Read the model definition and answer for the solid it produces. Units are mm, in the model's axes. A direction names the side the tool comes from. Give positions to 0.01 mm unless a question says otherwise; leave off trailing zeros. Write each loop counter-clockwise with the first axis right and the second up, starting at its lowest first coordinate (ties: lowest second). Pieces come first, ordered by that corner, then holes. Notation, with made-up numbers: (4.25, -38.5) -> (45.25, -38.5) arc R19 ccw to (45.25, -6.5) -> close; hole circle Ø3 at (82, 57). An arc over 180 degrees is marked (long way). Put each result on its own line as item: value. Start each with the question number.
from build123d import *

# Parameters (mm, degrees)
EXTRUDE_3_DEPTH           = 180
EXTRUDE_4_DEPTH           = 2
EXTRUDE_5_DEPTH           = 180
CUT_EXTRUDE_8_DEPTH       = 6
CUT_EXTRUDE_8_DEPTH_BACK  = 14
SKETCH_10_R               = 5
SKETCH_10_R_2             = 6
CUT_EXTRUDE_9_DEPTH       = 180
SKETCH_11_W               = 274.631033311
SKETCH_11_H               = 184
SKETCH_11_W_2             = 270.631033311
SKETCH_11_H_2             = 180
EXTRUDE_1_DEPTH           = 100
EXTRUDE_START             = -2
EXTRUDE_6_DEPTH           = 92
EXTRUDE_12_DEPTH          = 2
MIRROR_6_COPY_1_DEPTH     = 2
MIRROR_6_COPY_2_DEPTH     = 2
EXTRUDE_13_DEPTH          = 180
SKETCH_19_R               = 5
SKETCH_19_R_2             = 6
CUT_EXTRUDE_10_DEPTH      = 10
CUT_EXTRUDE_START         = -10
SKETCH_20_R               = 5
CUT_EXTRUDE_11_DEPTH      = 10
SKETCH_21_R               = 2
CUT_EXTRUDE_12_DEPTH      = 10
CUT_EXTRUDE_13_DEPTH      = 550.919994181
CUT_EXTRUDE_13_DEPTH_BACK = 550.919994181
SKETCH_22_R               = 2.5


with BuildPart() as part:
    # 草图1 → 凸台-拉伸3 (new body)
    with BuildSketch(Plane.XY):
        with BuildLine():
            Line((300, 0), (0, 0))
            Line((0, 0), (0, 200))
            Line((0, 200), (270, 200))
            Line((270, 200), (244.977927003, 106.616352266))
            ThreePointArc((244.977927003, 106.616352266), (245.721361032, 105.440582458), (246.409490454, 104.231613188))
            Line((246.409490454, 104.231613188), (272.606450746, 202))
            Line((272.606450746, 202), (-2, 202))
            Line((-2, 202), (-2, -2))
            Line((-2, -2), (302, -2))
            Line((302, -2), (302, 51.154700538))
            Line((302, 51.154700538), (248.866473036, 81.831356634))
            ThreePointArc((248.866473036, 81.831356634), (248.571049064, 80.851494363), (248.242374569, 79.882278975))
            Line((248.242374569, 79.882278975), (300, 50))
            Line((300, 50), (300, 0))
        make_face()
    extrude(amount=EXTRUDE_3_DEPTH)

    # 草图7 → 凸台-拉伸4 (add)
    with BuildSketch(Plane(origin=(0, 0, 0), x_dir=(-1, 0, 0), z_dir=(0, 0, -1))):
        Polygon((-272.606450746, 68.125074113), (-275.433236518, 66.493028586), (-302, 51.154700538), (-302, -2), (2, -2), (2, 202), (-272.606450746, 202), align=None)
    extrude_4 = extrude(amount=EXTRUDE_4_DEPTH)

    # 镜向5: 凸台-拉伸4 across plane
    add(extrude_4.mirror(Plane.XY.offset(90)))

    # 草图8 → 凸台-拉伸5 (add)
    with BuildSketch(Plane.XY):
        with BuildLine():
            Line((191.022225211, 97.764571353), (0, 144.327661976))
            Line((0, 144.327661976), (0, 140.399780569))
            Line((0, 140.399780569), (190.270548779, 94.019916677))
            ThreePointArc((190.270548779, 94.019916677), (190.586734182, 95.904218314), (191.022225211, 97.764571353))
        make_face()
    extrude(amount=EXTRUDE_5_DEPTH)

    # 草图10 → 切除-拉伸8 (cut, two sides: drawn at the far end of the back side and taken through both)
    with BuildSketch(Plane.XY.offset(-CUT_EXTRUDE_8_DEPTH_BACK)):
        with Locations(Location((60, 60, 0), (0, 0, 180))):
            Circle(SKETCH_10_R)
        with Locations(Location((95, 60, 0), (0, 0, 180))):
            Circle(SKETCH_10_R_2)
    extrude(amount=CUT_EXTRUDE_8_DEPTH + CUT_EXTRUDE_8_DEPTH_BACK, mode=Mode.SUBTRACT)

    # 草图8<3> → 切除-拉伸9 (cut)
    with BuildSketch(Plane.XY):
        Polygon((0, 200), (270, 200), (270.631033311, 202), (0, 202), align=None)
    extrude(amount=CUT_EXTRUDE_9_DEPTH, mode=Mode.SUBTRACT)

    # 草图11 → 拉伸-薄壁1 (add)
    with BuildSketch(Plane(origin=(0, 202, 0), x_dir=(1, 0, 0), z_dir=(0, 1, 0))):
        with Locations((135.315516656, -90)):
            Rectangle(SKETCH_11_W, SKETCH_11_H)
        with Locations((135.315516656, -90)):
            Rectangle(SKETCH_11_W_2, SKETCH_11_H_2, mode=Mode.SUBTRACT)
    extrude(amount=EXTRUDE_1_DEPTH)

    # 草图12 → 凸台-拉伸6 (add)
    with BuildSketch(Plane(origin=(0, 0, 180), x_dir=(-1, 0, 0), z_dir=(0, 0, -1)).offset(EXTRUDE_START)):
        Polygon((-98.869083806, 422), (-96.869083806, 422), (-15, 302), (-17, 302), align=None)
        Polygon((83.869083806, 422), (81.869083806, 422), (0, 302), (2, 302), align=None)
    extrude_6 = extrude(amount=EXTRUDE_6_DEPTH)

    # 草图16 → 凸台-拉伸12 (add)
    with BuildSketch(Plane.XY.offset(182)):
        Polygon((-83.869083806, 422), (98.869083806, 422), (17, 302), (-2, 302), align=None)
    extrude_12 = extrude(amount=-EXTRUDE_12_DEPTH)

    # 镜向6: 凸台-拉伸6 across plane
    add(extrude_6.mirror(Plane.XY.offset(90)))

    # 镜向6 copy 1 sketch → 镜向6 copy 1 (add)
    with BuildSketch(Plane(origin=(0, 0, 0), x_dir=(-1, 0, 0), z_dir=(0, 0, -1))):
        Polygon((-272.606450746, 68.125074113), (-275.433236518, 66.493028586), (-302, 51.154700538), (-302, -2), (2, -2), (2, 202), (-272.606450746, 202), align=None)
    extrude(amount=MIRROR_6_COPY_1_DEPTH)

    # 镜向6 copy 2 sketch → 镜向6 copy 2 (add)
    with BuildSketch(Plane(origin=(0, 0, 180), x_dir=(-1, 0, 0), z_dir=(0, 0, 1))):
        Polygon((-272.606450746, -68.125074113), (-275.433236518, -66.493028586), (-302, -51.154700538), (-302, 2), (2, 2), (2, -202), (-272.606450746, -202), align=None)
    extrude(amount=MIRROR_6_COPY_2_DEPTH)

    # 镜向7: 凸台-拉伸12 across plane
    add(extrude_12.mirror(Plane.XY.offset(90)))

    # 草图17 → 凸台-拉伸13 (add)
    with BuildSketch(Plane(origin=(0, 0, 180), x_dir=(-1, 0, 0), z_dir=(0, 0, -1))):
        Polygon((-15, 302), (-15, 252), (-10, 232.268619303), (-11.900860885, 231.877388977), (-17, 252), (-17, 300), (-270.631033311, 300), (-270.631033311, 302), (-17, 302), align=None)
    extrude(amount=EXTRUDE_13_DEPTH)

    # 草图19 → 切除-拉伸10 (cut)
    with BuildSketch(Plane.XY):
        with Locations((60, 60)):
            Circle(SKETCH_19_R)
        with Locations((95, 60)):
            Circle(SKETCH_19_R_2)
        with Locations((220, 90)):
            Circle(SKETCH_19_R)
    extrude(amount=-CUT_EXTRUDE_10_DEPTH, mode=Mode.SUBTRACT)

    # 草图20 → 切除-拉伸11 (cut)
    with BuildSketch(Plane(origin=(0, 0, 180), x_dir=(-1, 0, 0), z_dir=(0, 0, -1)).offset(CUT_EXTRUDE_START)):
        with Locations(Location((-220, 90, 0), (0, 0, 180))):
            Circle(SKETCH_20_R)
    extrude(amount=CUT_EXTRUDE_11_DEPTH, mode=Mode.SUBTRACT)

    # 草图21 → 切除-拉伸12 (cut)
    with BuildSketch(Plane(origin=(203.845281163, -54.620178469, 0), x_dir=(0, 0, -1), z_dir=(0.9659258262890673, -0.25881904510252457, 0))):
        with Locations(Location((-105, 174.455476118, 0), (0, 0, 90))):
            Circle(SKETCH_21_R)
        with Locations(Location((-75, 174.455476118, 0), (0, 0, 90))):
            Circle(SKETCH_21_R)
    extrude(amount=-CUT_EXTRUDE_12_DEPTH, mode=Mode.SUBTRACT)

    # 草图22 → 切除-拉伸13 (cut, two sides: drawn at the far end of the back side and taken through both)
    with BuildSketch(Plane.XY.offset(-CUT_EXTRUDE_13_DEPTH_BACK)):
        with Locations((28, 12.5)):
            Circle(SKETCH_22_R)
        with Locations((78, 12.5)):
            Circle(SKETCH_22_R)
        with Locations((128, 12.5)):
            Circle(SKETCH_22_R)
        with Locations((178, 12.5)):
            Circle(SKETCH_22_R)
        with Locations((228, 12.5)):
            Circle(SKETCH_22_R)
    extrude(amount=CUT_EXTRUDE_13_DEPTH + CUT_EXTRUDE_13_DEPTH_BACK, mode=Mode.SUBTRACT)


solid = part.part
1) A cutting plane is placed at D-D on y = 34.5. Give the vertices of the cut face in (x, z), and give its area (3 significant figures).
2) For a pull along Y with two mould halves and no side action, classify faces 5 (the face through (15, 277, 91)), 6 (the face through (89, 60, -1)), 7 (the face through (-41.51, 362.84, 91.26)) as pulls with the +Y half, pulls with the -Y half, needs draft (parallel to the pull), parting line crosses it, or undercut.
3) Each of these flat-tipped pins is pushed along its axis until it touches: pin 1 Ø1 at (x, z) = (67.5, 115) entering from +Y (3 decimals); pin 2 Ø24 at (y, z) = (282.5, 46) entering from +X; pin 3 Ø8 at (x, z) = (74.5, 63.5) entering from +Y; pin 4 Ø4 at (x, y) = (28, 12.5) entering from -Z. Where does it stop, or does it pass through?
4) A cutting plane is placed at A-A on x = 60. Give the vertices of the cut face in (y, z).
5) A cutting plane is placed at C-C on x = 220. Give the vertices of the cut face in (y, z).
6) Straight lines are drawn through the part: line 1 (X direction, y = 12.5, z = -1.05); line 2 (X direction, y = 255.5, z = 30); line 3 (X direction, y = 12, z = -1). For each, find the intervals that lie inside material, in ascending order. Write a range as [from, to].
7) For faces 1 (the face through (259.325, 152.431, 88.74)), 2 (the face through (57.36, 361.16, 88.71)), 3 (the face through (106, 161, 180)), 4 (the face through (12.535, 242.272, 91.26)), determine the directions among +Z, -Z, +X, -X, +Y, -Y from which every point of the face is accessible in a straight line to the end or side of a thin tool.
Results found:
1. outline: (-2, -2) -> (302, -2) -> (302, 182) -> (-2, 182) -> close; hole (0, 0) -> (300, 0) -> (300, 180) -> (0, 180) -> close
1. area: 1,940 mm²
2. face 5: needs draft
2. face 6: undercut
2. face 7: pulls with the +Y half
3. pin 1: stops at y = 379.685
3. pin 2: stops at x = 272.63
3. pin 3: stops at y = 395.08
3. pin 4: passes through
4. outline: (-2, -2) -> (55, -2) -> (55, 0) -> (0, 0) -> (0, 180) -> (125.77, 180) -> (125.77, 0) -> (65, 0) -> (65, -2) -> (302, -2) -> (302, 182) -> (-2, 182) -> close; (365.03, -2) -> (422, -2) -> (422, 0) -> (367.96, 0) -> (367.96, 180) -> (422, 180) -> (422, 182) -> (365.03, 182) -> close; hole (129.7, 0) -> (300, 0) -> (300, 180) -> (129.7, 180) -> close
5. outline: (-2, -2) -> (85, -2) -> (85, 0) -> (0, 0) -> (0, 180) -> (85, 180) -> (85, 182) -> (-2, 182) -> close; (95, -2) -> (302, -2) -> (302, 182) -> (95, 182) -> (95, 180) -> (300, 180) -> (300, 0) -> (95, 0) -> close
6. line 1: x = [-2, 25.5], [30.5, 75.5], [80.5, 125.5], [130.5, 175.5], [180.5, 225.5], [230.5, 302]
6. line 2: x = [-2, 0], [15, 17], [270.63, 272.63]
6. line 3: x = [-2, 25.55], [30.45, 75.55], [80.45, 125.55], [130.45, 175.55], [180.45, 225.55], [230.45, 302]
7. face 1: +X
7. face 2: +Z, -Z, +X
7. face 3: none
7. face 4: +Y
